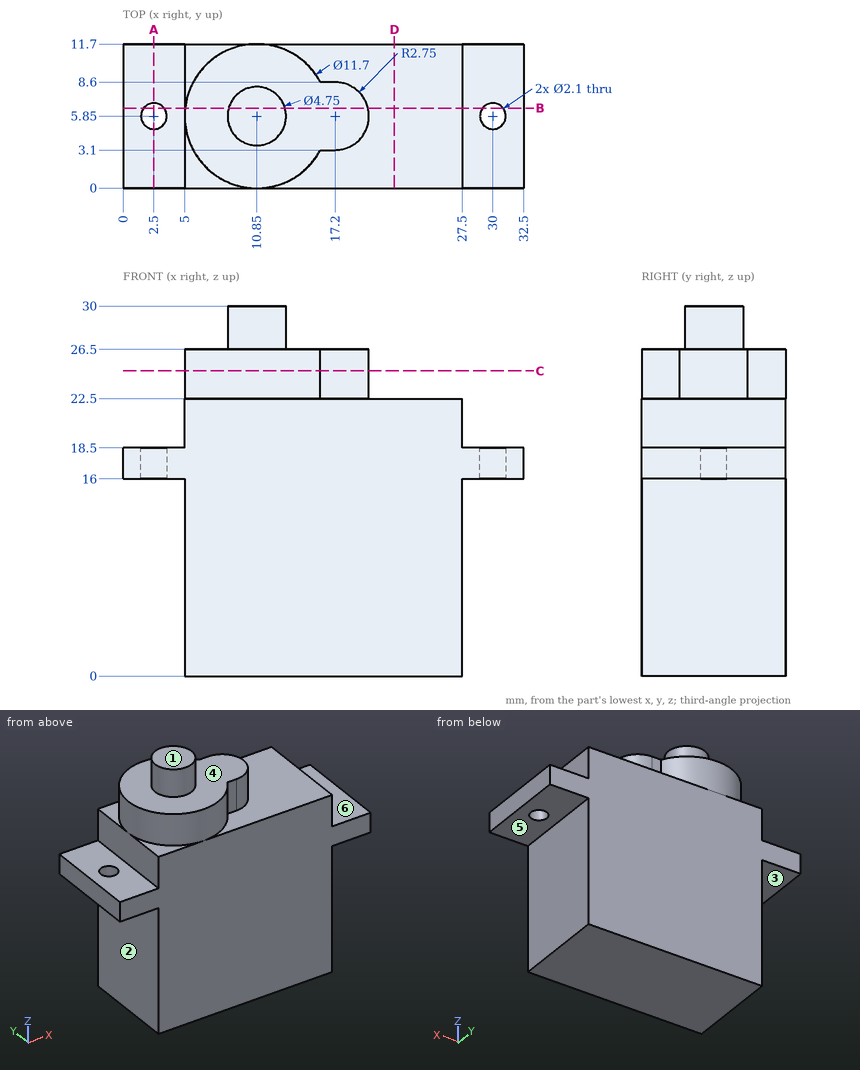
Geometry: see drawing. Coordinates: mm, zero at the bounding-box minimum. A direction names the side the tool comes from. Coordinates: 2 decimals unless noted, no trailing zeros. Write each loop counter-clockwise with the first axis right and the second up, starting at its lowest first coordinate (ties: lowest second). Pieces come first, ordered by that corner, then holes.
1) Section A-A on x = 2.5. Output: boundary loops of the cut face in (y, z), and give its area (3 significant figures).
2) Mould query, pull axis Z, two halves, no side actions, for the marked faces 1, 2 and 3. Classes: pulls with the +Z half, pulls with the -Z half, needs draft (parallel to the pull), parting line crosses it, or undercut.
3) Material intervals for line 1 along Y through (x, z) = (30, 17.55); line 2 along Z through (x, y) = (26.5, 3); line 3 along X through (y, z) = (7.75, 1.5), sorted ascending.
4) Pin query (flat end, axial travel): pin 1 Ø3.5 at (x, y) = (2.5, 5.85) entering from +Z; pin 2 Ø1.5 at (x, y) = (29.5, 7) entering from -Z; pin 3 Ø6 at (y, z) = (3.5, 10.5) entering from -X. Return the tip coordinate at first contact, or that it passes through.
5) Section B-B on y = 6.5. State how many separate pieces and enclosed holes the cut face has, and give its area (3 significant figures).
6) Section D-D on x = 22. Output: boundary loops of the cut face in (y, z), and give its area (3 significant figures).
7) Set-up query: the marked faces 4, 5 and 6. Return all of +Z, -Z, +X, -X, +Y, -Y with unobstructed straight access to the full face (end or side cutting, diameter ignored); none if empty.
8) Section C-C on z = 24.75. Output: boundary loops of the cut face in (x, y), and give its area (3 significant figures).
Check result:
1. outline: (0, 16) - (4.8, 16) - (4.8, 18.5) - (0, 18.5) - close; (6.9, 16) - (11.7, 16) - (11.7, 18.5) - (6.9, 18.5) - close
1. area: 24.0 mm2
2. face 1: pulls with the +Z half
2. face 2: needs draft
2. face 3: pulls with the -Z half
3. line 1: y = 0 to 4.8, 6.9 to 11.7
3. line 2: z = 0 to 22.5
3. line 3: x = 5 to 27.5
4. pin 1: stops at z = 18.5
4. pin 2: stops at z = 16
4. pin 3: stops at x = 5
5. separate pieces: 3
5. enclosed holes: 0
5. area: 598 mm2
6. outline: (0, 0) - (11.7, 0) - (11.7, 22.5) - (0, 22.5) - close
6. area: 263 mm2
7. face 4: +Z
7. face 5: -Z, +X, +Y, -Y
7. face 6: +Z, +X, +Y, -Y
8. outline: (16.01, 3.1) - (17.2, 3.1) arc R2.75 ccw to (17.2, 8.6) - (16.01, 8.6) arc R5.85 ccw (long way) to start
8. area: 123 mm2
